Study the drawing (mm; zero at the part's minimum x, y, z) and answer. A direction names the side the tool comes from. Give positions to 0.01 mm unless a question says otherwise; leave off trailing zeros. Write each loop counter-clockwise with the first axis right and the second up, starting at its lowest first coordinate (ties: lowest second). Pieces come first, ordered by that corner, then holes.
1) Find section D-D (z = 33.5). Determine the outline of the cut face in (x, y).
2) Find section B-B (x = 8.5). Determine the outline of the cut face in (y, z), plus the area to 3 significant figures.
3) Determine the mould class of the marked faces 4, 5 and 6 for opening direction Z: pulls with the +Z half, pulls with the -Z half, needs draft (parallel to the pull), parting line crosses it, or undercut.
4) Given pin 1 Ø5 at (x, z) = (13, 44) entering from +Y; pin 2 Ø5 at (y, z) = (10, 30) entering from -X; pin 3 Ø2 at (x, y) = (15, 5) entering from -Z, each flat-ended and moving along its own axis, determine where each tip first touches the part or whether it passes through.
5) Straight lines are drawn through the part: probe 1 along Y at (x, z) = (25, 5.5); probe 2 along Y at (x, z) = (15, 5.5); probe 3 along Z at (x, y) = (7.5, 33). For each, find the intervals that lie inside material, in ascending order.
6) Find section A-A (y = 30). Determine the outline of the cut face in (x, z).
7) A tool of negligible diameter and unlimited length cuts with its end or side. For the marked faces 1, 2 and 3, from which of +Z, -Z, +X, -X, +Y, -Y can it reach the whole face along a straight path? Write none if from no direction.
8) Find section C-C (y = 15). Determine the outline of the cut face in (x, z).
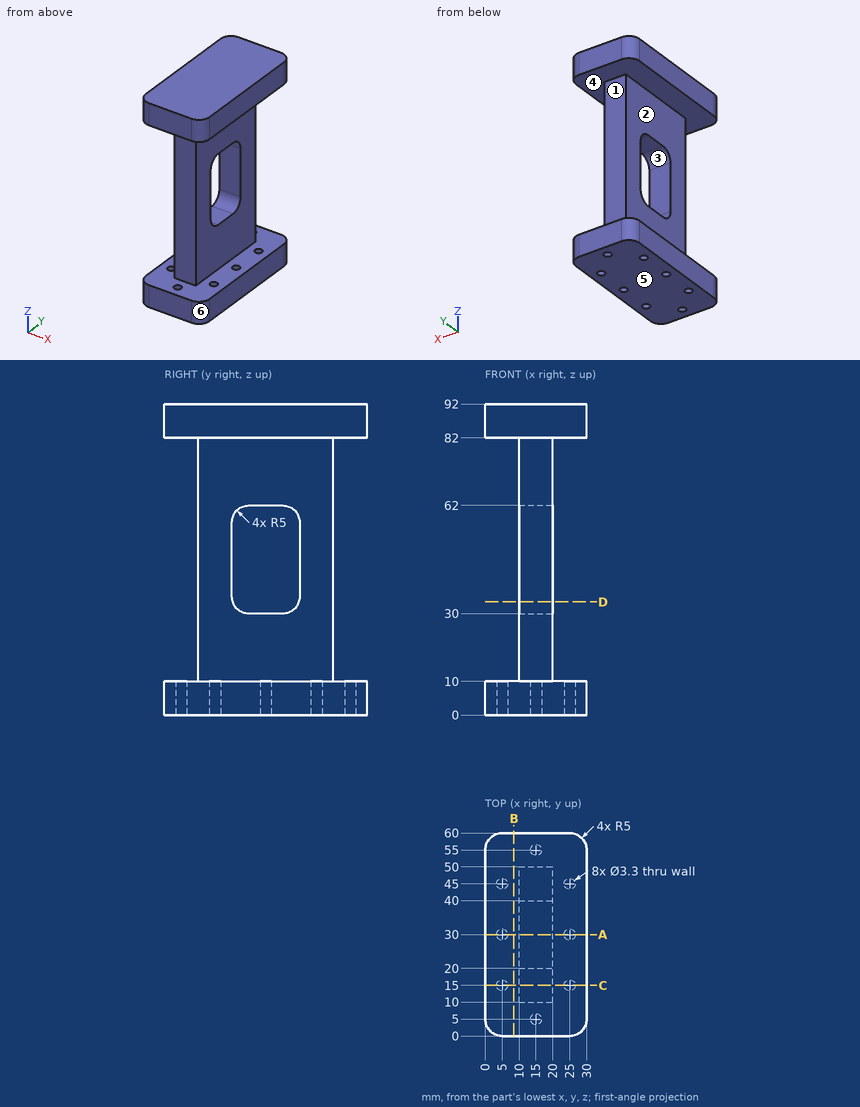
Results:
1. outline: (10, 10) - (20, 10) - (20, 20.23) - (10, 20.23) - close; (10, 39.77) - (20, 39.77) - (20, 50) - (10, 50) - close
2. outline: (0, 0) - (60, 0) - (60, 10) - (0, 10) - close; (0, 82) - (60, 82) - (60, 92) - (0, 92) - close
2. area: 1,200 mm2
3. face 4: undercut
3. face 5: pulls with the -Z half
3. face 6: needs draft
4. pin 1: stops at y = 50
4. pin 2: stops at x = 10
4. pin 3: stops at z = 82
5. probe 1: y = 0 to 13.35, 16.65 to 28.35, 31.65 to 43.35, 46.65 to 60
5. probe 2: y = 0 to 3.35, 6.65 to 53.35, 56.65 to 60
5. probe 3: z = 0 to 10, 82 to 92
6. outline: (0, 0) - (3.35, 0) - (3.35, 10) - (0, 10) - close; (0, 82) - (10, 82) - (10, 62) - (20, 62) - (20, 82) - (30, 82) - (30, 92) - (0, 92) - close; (6.65, 0) - (23.35, 0) - (23.35, 10) - (20, 10) - (20, 30) - (10, 30) - (10, 10) - (6.65, 10) - close; (26.65, 0) - (30, 0) - (30, 10) - (26.65, 10) - close
7. face 1: +X, -X, +Y
7. face 2: -X, +Y, -Y
7. face 3: +X, -X
8. outline: (0, 0) - (3.35, 0) - (3.35, 10) - (0, 10) - close; (0, 82) - (10, 82) - (10, 10) - (6.65, 10) - (6.65, 0) - (23.35, 0) - (23.35, 10) - (20, 10) - (20, 82) - (30, 82) - (30, 92) - (0, 92) - close; (26.65, 0) - (30, 0) - (30, 10) - (26.65, 10) - close
